from build123d import *

# Parameters (mm, degrees)
SKETCH006_W                 = 14
SKETCH006_H                 = 14
PAD002_DEPTH                = 3
POCKET004_DEPTH             = 2
SKETCH008_R                 = 0.9
POCKET005_DEPTH             = 1.001
CLONE001007_PLACEMENT_ANGLE = 90
PAD_DEPTH                   = 3
SKETCH010_W                 = 12
SKETCH010_H                 = 12
POCKET_DEPTH                = 2
CLONE001006_PLACEMENT_ANGLE = 180
FILLET001_R                 = 2
CLONE001009_PLACEMENT_ANGLE = -90
CLONE001012_PLACEMENT_ANGLE = 180


with BuildPart() as obj1:
    # Sketch006 → Pad002 (new body)
    with BuildSketch(Plane.XY):
        Rectangle(SKETCH006_W, SKETCH006_H)
    extrude(amount=PAD002_DEPTH)

    # Sketch007 → Pocket004 (cut)
    with BuildSketch(Plane.XY.offset(3)):
        with BuildLine():
            Line((-3, 7), (-3, 4.963869))
            ThreePointArc((-3, 4.963869), (-5.8, 0), (-3, -4.963869))
            Line((-3, -7), (-3, -4.963869))
            Line((3, -7), (-3, -7))
            Line((3, -4.963869), (3, -7))
            ThreePointArc((3, -4.963869), (5.8, 0), (3, 4.963869))
            Line((3, 7), (3, 4.963869))
            Line((-3, 7), (3, 7))
        make_face()
    extrude(amount=-POCKET004_DEPTH, mode=Mode.SUBTRACT)

    # Sketch008 → Pocket005 (cut, through all)
    with BuildSketch(Plane.XY.offset(1)):
        Circle(SKETCH008_R)
    extrude(amount=-POCKET005_DEPTH, mode=Mode.SUBTRACT)


with BuildPart() as obj1_1:
    # Clone001005 placement: moved
    add(obj1.part.moved(Location((14, 0, 0))))


with BuildPart() as obj2:
    # Clone001007 base: copy of obj1
    add(obj1_1.part)


with BuildPart() as obj2_1:
    # Clone001007 placement: moved
    add(obj2.part.moved(Location((0, -28, 0))).rotate(Axis((0, -28, 0), (0, 0, 1)), CLONE001007_PLACEMENT_ANGLE))


with BuildPart() as obj3:
    # Sketch → Pad (new body)
    with BuildSketch(Plane.XY):
        Polygon((-7, -7), (-7, 7), (7, 7), (7, 5), (-5, -7), align=None)
    extrude(amount=PAD_DEPTH)

    # Sketch010 → Pocket (cut)
    with BuildSketch(Plane(origin=(0, 0, 0), x_dir=(1, 0, 0), z_dir=(0, 0, -1))):
        with Locations((1, 1)):
            Rectangle(SKETCH010_W, SKETCH010_H)
    extrude(amount=-POCKET_DEPTH, mode=Mode.SUBTRACT)


with BuildPart() as obj3_1:
    # Clone001006 placement: moved
    add(obj3.part.rotate(Axis((0, 0, 0), (0, 0, 1)), CLONE001006_PLACEMENT_ANGLE))


with BuildPart() as clone_of_corner_holder_double002:
    # Fusion001 base: copy of obj1
    add(obj1_1.part)

    # Fusion001: union obj2, obj3
    add(obj2_1.part)
    add(obj3_1.part)

    # Fillet001
    fillet001_edges = [clone_of_corner_holder_double002.edges().sort_by_distance(p)[0] for p in [
        (21, 7, 1.5),
        (21, -7, 1.5),
        (7, -21, 1.5),
        (-7, -21, 1.5),
    ]]
    fillet(fillet001_edges, radius=FILLET001_R)


with BuildPart() as clone_of_corner_holder_double002_1:
    # Clone001008 placement: moved
    add(clone_of_corner_holder_double002.part.moved(Location((-13.497608, 48.033168, 0))))


with BuildPart() as clone_of_corner_holder_double002_2:
    # Clone001009 placement: moved
    add(clone_of_corner_holder_double002_1.part.moved(Location((-30.900794, -30.494573, 0))).rotate(Axis((-30.900794, -30.494573, 0), (0, 0, 1)), CLONE001009_PLACEMENT_ANGLE))


with BuildPart() as clone_of_corner_holder_double002_3:
    # Clone001012 placement: moved
    add(clone_of_corner_holder_double002_2.part.moved(Location((84.263711, 16.007107, 0))).rotate(Axis((84.263711, 16.007107, 0), (0, 0, 1)), CLONE001012_PLACEMENT_ANGLE))


with BuildPart() as clone_of_corner_holder_double002_4:
    # Clone001018 placement: moved
    add(clone_of_corner_holder_double002_3.part.moved(Location((-42.131337, -8.004072, 63))))


solid = clone_of_corner_holder_double002_4.part
The model under review builds one solid part; all positions refer to its coordinate system, in mm. A direction names the side the tool comes from. Coordinates: 2 decimals unless noted, no trailing zeros. Write each loop counter-clockwise with the first axis right and the second up, starting at its lowest first coordinate (ties: lowest second). Pieces come first, ordered by that corner, then holes. Notation, with made-up numbers: (83, -24) -> (127, -24) arc R30 ccw to (127, 6) -> close; hole circle Ø3 at (11.5, 31). An arc over 180 degrees is marked (long way). Answer in a Markdown table with one row per item.
1. Wall thickness on probe 1 along X at (y, z) = (25, 63.7); probe 2 along X at (y, z) = (39, 63.5): over which ranges is each line inside the solid? List them lowest first. Write a range as [from, to].
Answers below:
| item | result |
|---|---|
| probe 1 | x = [30, 38.1], [39.9, 46] |
| probe 2 | x = [18, 24.1], [25.9, 32] |
2. We need section A-A, the plane z = 64.5. State the section outline as (x, y) points.
Answers below:
| item | result |
|---|---|
| outline | (18, 30) -> (30, 30) -> (30, 18) -> (36, 18) -> (36, 20.04) arc R5.8 cw to (36, 29.96) -> (36, 32) -> (32, 32) -> (32, 36) -> (29.96, 36) arc R5.8 cw to (20.04, 36) -> (18, 36) -> close; (18, 42) -> (20.04, 42) arc R5.8 cw to (29.96, 42) -> (32, 42) -> (32, 44) arc R2 ccw to (30, 46) -> (20, 46) arc R2 ccw to (18, 44) -> close; (42, 18) -> (44, 18) arc R2 ccw to (46, 20) -> (46, 30) arc R2 ccw to (44, 32) -> (42, 32) -> (42, 29.96) arc R5.8 cw to (42, 20.04) -> close |
3. Draft analysis for pull direction X (two halves, no side actions). For faces 1 (the flat face through (45, 25, 66)), 2 (the cylindrical face through (45.43, 31.4, 64.52)), 3 (the flat face through (24.9, 37.6, 64)), state which applies: +X half, -X half, draft (parallel to the pull), parting line (faces both ways), or undercut.
Answers below:
| item | result |
|---|---|
| face 1 | draft |
| face 2 | +X half |
| face 3 | undercut |
4. We need section B-B, the plane x = 25. State the section outline as (y, z) points, and give its area (3 significant figures).
Answers below:
| item | result |
|---|---|
| outline | (23, 65) -> (30, 65) -> (30, 63) -> (38.1, 63) -> (38.1, 64) -> (33.2, 64) -> (33.2, 66) -> (23, 66) -> close; (39.9, 63) -> (46, 63) -> (46, 66) -> (44.8, 66) -> (44.8, 64) -> (39.9, 64) -> close |
| area | 30.0 mm^2 |
5. We need section D-D, the plane y = 43. State the section outline as (x, z) points.
Answers below:
| item | result |
|---|---|
| outline | (18, 63) -> (32, 63) -> (32, 66) -> (29.2, 66) -> (29.2, 64) -> (20.8, 64) -> (20.8, 66) -> (18, 66) -> close |
6. For faces 4 (the flat face through (31, 36, 65)), 5 (the flat face through (38.1, 32, 63.8)), 6 (the flat face through (42, 31, 65)), 7 (the flat face through (40.4, 24.9, 64)), list the 3-axis set-ups (+Z, -Z, +X, -X, +Y, -Y) from which the entire face can be reached by the end or side of a thin tool; tool diameter is ignored.
Answers below:
| item | result |
|---|---|
| face 4 | +Z, +X, -X |
| face 5 | +Z, -Z, +X, +Y |
| face 6 | +Z, +Y, -Y |
| face 7 | +Z |
7. Clearance check with flat-ended pins moving along their axes: pin 1 Ø0.6 at (y, z) = (25.5, 64) entering from -X; pin 2 Ø0.6 at (y, z) = (19.5, 64.5) entering from +X; pin 3 Ø6 at (x, y) = (24, 41.5) entering from +Z. State where each tip first meets the part, or that it passes through.
Answers below:
| item | result |
|---|---|
| pin 1 | stops at x = 30 |
| pin 2 | stops at x = 45.99 |
| pin 3 | stops at z = 64 |
